Autodesk Inventor part; units mm, degrees
ref_plane "YZ Plane" through (0, 0, 0) normal (1, 0, 0) x (0, 1, 0)
ref_plane "XZ Plane" through (0, 0, 0) normal (0, 1, 0) x (-1, 0, 0)
ref_plane "XY Plane" through (0, 0, 0) normal (0, 0, 1) x (1, 0, 0)
sketch "Skizze1" plane through (0, 0, 0) normal (0, 1, 0) x (-1, 0, 0)
  line L0 (20, 10) -> (-20, 10)
  line L1 (-20, 10) -> (-20, -10)
  line L2 (-20, -10) -> (20, -10)
  line L3 (20, -10) -> (20, 10)
  line L4 (20, 10) -> (-20, -10) construction
  line L5 (-20, 10) -> (20, -10) construction
  point P0 (0, 0)
  dimension "d0" = 40
  dimension "d1" = 20
extrude "Extrusion1" add sketch "Skizze1" along normal blind 20
sketch "Skizze2" plane through (20, 0, 10) normal (1, 0, 0) x (0, 0, -1)
  circle A0 centre (10, 10) radius 2.5
  line L0 (0, 20) -> (20, 20)
  line L1 (0, 0) -> (20, 0)
  line L2 (20, 0) -> (20, 20)
  line L3 (0, 0) -> (0, 20)
  point P0 (10, 0)
  dimension "d4" = 5
  dimension "d5" = 10
  dimension "d6" = 10
  dimension "d7" = 10
  dimension "d8" = 10
hole "Bohrung1" at (20, 10, 0) direction (-1, 0, 0) diameter 4 end through all
equation "\"d5\" = d6"
equation "\"d7\" = d8"
properties part number "Z-Joint"
Input: part model. Units: mm. Frame: model coordinates. Give positions to 0.01 mm unless a question says otherwise; leave off trailing zeros. Loops run counter-clockwise (first coordinate to the right, second up) from the corner with the lowest first, then second, coordinate; pieces in that order, holes last. Notation, with made-up numbers: M 38,88 L 90,88 A14 cw 90,95 Z; hole C 61.5,-38 d2. An arc over 180 degrees is marked long. Use one line per item in the form item = value.
1. Line query: L1, parallel to Y at x = 5.5, z = 0; L2, parallel to Z at x = -8.5, y = 10; L3, parallel to Z at x = 13, y = 11. Output: solid intervals per line, ascending.
Numbers:
L1 = 0 to 8, 12 to 20
L2 = -10 to -2, 2 to 10
L3 = -10 to -1.73, 1.73 to 10
2. Section query A-A, the plane z = 0. Return the cut outline in (x, y), and give its area (3 significant figures).
Numbers:
outline = M -20,0 L 20,0 L 20,8 L -20,8 Z; M -20,12 L 20,12 L 20,20 L -20,20 Z
area = 640 mm²
3. Section query B-B, the plane x = -13. Return the cut outline in (y, z), and give its area (3 significant figures).
Numbers:
outline = M 0,-10 L 20,-10 L 20,10 L 0,10 Z; hole C 10,0 d4
area = 387 mm²
4. Section query C-C, the plane y = 11.5. Return the cut outline in (x, z).
Numbers:
outline = M -20,-10 L 20,-10 L 20,-1.32 L -20,-1.32 Z; M -20,1.32 L 20,1.32 L 20,10 L -20,10 Z
